Part model, mm, in its own coordinate system. Coordinates: 2 decimals unless noted, no trailing zeros.
```python
from build123d import *

# Parameters (mm, degrees)
SKETCH1_W              = 60
SKETCH1_H              = 200
BOSS_EXTRUDE1_DEPTH    = 5
SKETCH6_R              = 2
CUT_EXTRUDE3_DEPTH     = 5
SKETCH7_R              = 2
CUT_EXTRUDE4_DEPTH     = 5
LPATTERN1_COUNT        = 6
LPATTERN1_PITCH        = 23
CUT_EXTRUDE_1312_DEPTH = 5
CHAMFER_1373_SIZE      = 5


with BuildPart() as part:
    # Sketch1 → Boss-Extrude1 (new body)
    with BuildSketch(Plane.XY):
        with Locations((-30, 100)):
            Rectangle(SKETCH1_W, SKETCH1_H)
    extrude(amount=BOSS_EXTRUDE1_DEPTH)

    # Sketch6 → Cut-Extrude3 (cut)
    with BuildSketch(Plane.XY):
        with Locations((-8, 8)):
            Circle(SKETCH6_R)
        with Locations((-8, 20)):
            Circle(SKETCH6_R)
    cut_extrude3 = extrude(amount=CUT_EXTRUDE3_DEPTH, mode=Mode.SUBTRACT)

    # Mirror1: Cut-Extrude3 across plane
    add(cut_extrude3.mirror(Plane.ZX.offset(100)), mode=Mode.SUBTRACT)

    # Sketch7 → Cut-Extrude4 (cut)
    with BuildSketch(Plane.XY):
        with Locations((-8, 43)):
            Circle(SKETCH7_R)
    cut_extrude4 = extrude(amount=CUT_EXTRUDE4_DEPTH, mode=Mode.SUBTRACT)

    # LPattern1: Cut-Extrude4 ×6
    with Locations(*[(0, i * LPATTERN1_PITCH, 0) for i in range(1, LPATTERN1_COUNT)]):
        add(cut_extrude4, mode=Mode.SUBTRACT)

    # Sketch3 → Cut-Extrude 1312 (cut)
    with BuildSketch(Plane(origin=(-200, 0, 0), x_dir=(-1, 0, 0), z_dir=(0, 0, -1))):
        Polygon((-140, 0), (-175.265396142, 0), (-140, 200), align=None)
    extrude(amount=-CUT_EXTRUDE_1312_DEPTH, mode=Mode.SUBTRACT)

    # Chamfer 1373
    chamfer_1373_edges = [part.edges().sort_by_distance(p)[0] for p in [
        (-42.367301929, 100, 5),
    ]]
    chamfer(chamfer_1373_edges, length=CHAMFER_1373_SIZE - 0.0001)  # a hair under: the kernel refuses the full size


solid = part.part
```
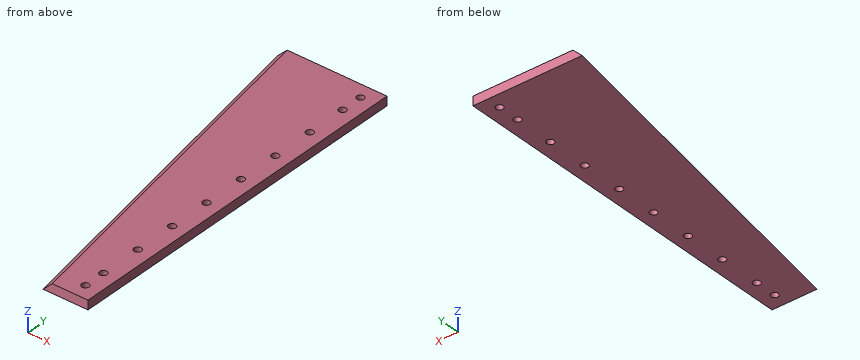
Q1. Saw through at B-B (z = 2.3). Count the separate pieces of the cut face and the enclosed holes in it, plus the area to 3 significant figures.
Q2. Probe line 1 (X direction, y = 180, z = 1.6); line 2 (X direction, y = 180, z = 2.4); line 3 (X direction, y = 35.5, z = 4.4). List the from-to ranges inside material, lowest first.
Q3. Drop flat-ended pins along their axis: P1, Ø4.5, axis at x = -8, y = 158, coming from the -Z side; P2, Ø2, axis at y = 83.5, z = 4.5, coming from the -X side. Give the stop position or say it passes through.
Checked values:
1. separate pieces: 1
1. enclosed holes: 10
1. area: 7,880 mm2
2. line 1: x = -54.85 to -10, -6 to 0
2. line 2: x = -54.04 to -10, -6 to 0
2. line 3: x = -26.53 to 0
3. P1: stops at z = 0
3. P2: stops at x = -35.92
